Here's how the part is built. I have some questions about the finished solid (model axes, mm). Give positions to 0.01 mm unless a question says otherwise; leave off trailing zeros. Loops run counter-clockwise (first coordinate to the right, second up) from the corner with the lowest first, then second, coordinate; pieces in that order, holes last. Notation, with made-up numbers: (-32.75, 66.25) - (20.25, 66.25) arc R26 ccw to (20.25, 85.25) - close; hole circle Ø4 at (27, 35.5). An arc over 180 degrees is marked (long way). Return JSON: item names as keys, results as strings. Group by question number.
(1) If we section it at B-B (z = 15.5): Please give me the cut outline in (x, y), then the cut area to 3 significant figures.
(2) I need wall thicknesses on probe 1 along X at (y, z) = (-0.35, 23.5); probe 2 along Z at (x, y) = (-27, -1.5); probe 3 along Z at (x, y) = (-37, -0.25). Which ranges of each line are inside material? Lowest first, please. Write a range as [from, to].
(3) If we section it at A-A (x = -37): State how many separate pieces and enclosed holes the cut face has, then the cut area to 3 significant figures.
(4) If we section it at D-D (y = -1.3): Please give me the cut outline in (x, z).
(5) For P1, Ø2.5, axis at x = -51.5, z = 17.76, coming from the -Y side, with a flat end and sliding along its axis, tell me the tip position at first contact or that it passes through.
(6) If we mould it in two halves opening along Z, with no side actions, what happens to faces 1 (the cylindrical face through (-38.19, -1.52, 11.85)), 2 (the flat face through (-32, -1, 32.527)), 3 (the flat face through (-64, -1, 16))? For each: released by +Z, released by -Z, zero draft, split by the parting line, or undercut.
```python
from build123d import *

# Parameters (mm, degrees)
F0_W     = 64
F0_H     = 32.527
F1_DEPTH = 3
F2_SIZE  = 2.99999
F6_D     = 6
F7_D     = 3


# Not quite as in the source:
# - a fillet or chamfer is up to 0.001 mm smaller than in the source, because OpenCascade refuses the exact size


with BuildPart() as f1:
    # F0 (on Front) → F1 (new body)
    with BuildSketch(Plane.XZ):
        with Locations((-32, 16.2635)):
            Rectangle(F0_W, F0_H)
    extrude(amount=F1_DEPTH)

    # F2 (size 3 in the source; OpenCascade refuses exactly that, so slightly less here)
    f2_edges = [f1.edges().sort_by_distance(p)[0] for p in [
        (-32, 0, 0),
    ]]
    chamfer(f2_edges, length=F2_SIZE)

    # F6 (through all)
    with Locations(Plane(origin=(0, 0, 0), x_dir=(-1, 0, 0), z_dir=(0, 1, 0))):
        with Locations((32, 17.7635)):
            Hole(F6_D / 2)

    # F7 (through all)
    with Locations(Plane(origin=(0, 0, 0), x_dir=(-1, 0, 0), z_dir=(0, 1, 0))):
        with Locations((37, 22.7635), (27, 22.7635), (27, 12.7635), (37, 12.7635), (12.5, 17.7635), (51.5, 17.7635)):
            Hole(F7_D / 2)


solid = f1.part
```
Values:
{
 "1": {"outline": "(-64, -3) - (-33.97, -3) - (-33.97, 0) - (-64, 0) - close; (-30.03, -3) - (0, -3) - (0, 0) - (-30.03, 0) - close", "area": "180 mm2"},
 "2": {"probe 1": "[-64, -38.31], [-35.69, -28.31], [-25.69, 0]", "probe 2": "[1.5, 11.26], [14.26, 21.26], [24.26, 32.53]", "probe 3": "[2.75, 11.26], [14.26, 21.26], [24.26, 32.53]"},
 "3": {"separate pieces": "3", "enclosed holes": "0", "area": "75.1 mm2"},
 "4": {"outline": "(-64, 1.7) - (0, 1.7) - (0, 32.53) - (-64, 32.53) - close; hole circle Ø3 at (-51.5, 17.76); hole circle Ø3 at (-37, 12.76); hole circle Ø3 at (-37, 22.76); hole circle Ø6 at (-32, 17.76); hole circle Ø3 at (-27, 12.76); hole circle Ø3 at (-27, 22.76); hole circle Ø3 at (-12.5, 17.76)"},
 "5": {"P1": "through"},
 "6": {"face 1": "undercut", "face 2": "released by +Z", "face 3": "zero draft"}
}
